Geometry: final body of the model. Coordinates: model frame, mm. Give positions to 0.01 mm unless a question says otherwise; leave off trailing zeros. Order: outer loops, then holes, each group sorted by start corner. A loop starts at its lowest first (then second) coordinate and runs counter-clockwise, first axis right, second up. Notation, with made-up numbers: (-20.75, -29.5) -> (34.25, -29.5) arc R8 ccw to (34.25, -20.5) -> close; hole circle Ø1 at (-1.5, 20.5). An arc over 180 degrees is marked (long way). One line per question, with ' | ' between items. Start each with the question number.
(1) Section C-C (z = 0.7). State how many separate pieces and enclosed holes the cut face has, then the cut area to 3 significant figures.
(2) Section A-A (y = 0). Return loops of the section in (x, z), then the cut area to 4 significant figures.
(3) Ray query, L1, parallel to Y at x = 0, z = -0.75; L2, parallel to X at y = -23.5, z = -1.15; L3, parallel to Y at x = -20, z = 0.9. Return the intervals inside material, ascending.
(4) First-contact query: pin 1 Ø6.5 at (x, y) = (-22.98, 22.98) entering from +Z; pin 2 Ø6.5 at (x, y) = (0, -45.75) entering from -Z; pin 3 Ø3 at (y, z) = (-35, 1.5) entering from +X. Flat tips, straight axial feed; report the tip coordinate or a pass-through.
(5) Section D-D (x = -15). Return loops of the section in (y, z), then the cut area to 3 significant figures.
```python
from build123d import *

# Parameters (mm, degrees)
SKETCH1_R           = 2.25
SKETCH1_R_2         = 22.5
BOSS_EXTRUDE1_DEPTH = 2.5
SKETCH3_R           = 4
CUT_EXTRUDE2_DEPTH  = 4
SKETCH4_R           = 4
CUT_EXTRUDE3_DEPTH  = 4


with BuildPart() as part:
    # Sketch1 → Boss-Extrude1 (new, symmetric)
    with BuildSketch(Plane.XY):
        with BuildLine():
            ThreePointArc((4.630966194, 47.635245902), (0, 50.75), (-4.630966194, 47.635245902))
            ThreePointArc((-4.630966194, 47.635245902), (-7.268500835, 43.914585958), (-11.283903543, 41.752078042))
            ThreePointArc((-11.283903543, 41.752078042), (-30.582368286, 30.582368286), (-41.752078042, 11.283903543))
            ThreePointArc((-41.752078042, 11.283903543), (-43.914585958, 7.268500835), (-47.635245902, 4.630966194))
            ThreePointArc((-47.635245902, 4.630966194), (-50.75, 0), (-47.635245902, -4.630966194))
            ThreePointArc((-47.635245902, -4.630966194), (-43.914585958, -7.268500835), (-41.752078042, -11.283903543))
            ThreePointArc((-41.752078042, -11.283903543), (-30.582368286, -30.582368286), (-11.283903543, -41.752078042))
            ThreePointArc((-11.283903543, -41.752078042), (-7.268500835, -43.914585958), (-4.630966194, -47.635245902))
            ThreePointArc((-4.630966194, -47.635245902), (0, -50.75), (4.630966194, -47.635245902))
            ThreePointArc((4.630966194, -47.635245902), (7.268500835, -43.914585958), (11.283903543, -41.752078042))
            ThreePointArc((11.283903543, -41.752078042), (30.582368286, -30.582368286), (41.752078042, -11.283903543))
            ThreePointArc((41.752078042, -11.283903543), (43.914585958, -7.268500835), (47.635245902, -4.630966194))
            ThreePointArc((47.635245902, -4.630966194), (50.75, 0), (47.635245902, 4.630966194))
            ThreePointArc((47.635245902, 4.630966194), (43.914585958, 7.268500835), (41.752078042, 11.283903543))
            ThreePointArc((41.752078042, 11.283903543), (30.582368286, 30.582368286), (11.283903543, 41.752078042))
            ThreePointArc((11.283903543, 41.752078042), (7.268500835, 43.914585958), (4.630966194, 47.635245902))
        make_face()
        with Locations((-45.75, 0)):
            Circle(SKETCH1_R, mode=Mode.SUBTRACT)
        with Locations((0, 45.75)):
            Circle(SKETCH1_R, mode=Mode.SUBTRACT)
        with Locations((45.75, 0)):
            Circle(SKETCH1_R, mode=Mode.SUBTRACT)
        with Locations((0, -45.75)):
            Circle(SKETCH1_R, mode=Mode.SUBTRACT)
        with Locations((-22.980970389, 22.980970389)):
            Circle(SKETCH1_R, mode=Mode.SUBTRACT)
        with Locations((22.980970389, 22.980970389)):
            Circle(SKETCH1_R, mode=Mode.SUBTRACT)
        with Locations((22.980970389, -22.980970389)):
            Circle(SKETCH1_R, mode=Mode.SUBTRACT)
        with Locations((-22.980970389, -22.980970389)):
            Circle(SKETCH1_R, mode=Mode.SUBTRACT)
        Circle(SKETCH1_R_2, mode=Mode.SUBTRACT)
    extrude(amount=BOSS_EXTRUDE1_DEPTH, both=True)

    # Sketch3 → Cut-Extrude2 (cut)
    with BuildSketch(Plane.XY.offset(2.5)):
        with Locations((-22.980970389, -22.980970389)):
            Circle(SKETCH3_R)
        with Locations((-22.980970389, 22.980970389)):
            Circle(SKETCH3_R)
        with Locations((22.980970389, 22.980970389)):
            Circle(SKETCH3_R)
        with Locations((22.980970389, -22.980970389)):
            Circle(SKETCH3_R)
    extrude(amount=-CUT_EXTRUDE2_DEPTH, mode=Mode.SUBTRACT)

    # Sketch4 → Cut-Extrude3 (cut)
    with BuildSketch(Plane(origin=(0, 0, -2.5), x_dir=(-1, 0, 0), z_dir=(0, 0, -1))):
        with Locations((0, 45.75)):
            Circle(SKETCH4_R)
        with Locations((45.75, 0)):
            Circle(SKETCH4_R)
        with Locations((0, -45.75)):
            Circle(SKETCH4_R)
        with Locations((-45.75, 0)):
            Circle(SKETCH4_R)
    extrude(amount=-CUT_EXTRUDE3_DEPTH, mode=Mode.SUBTRACT)


solid = part.part
```
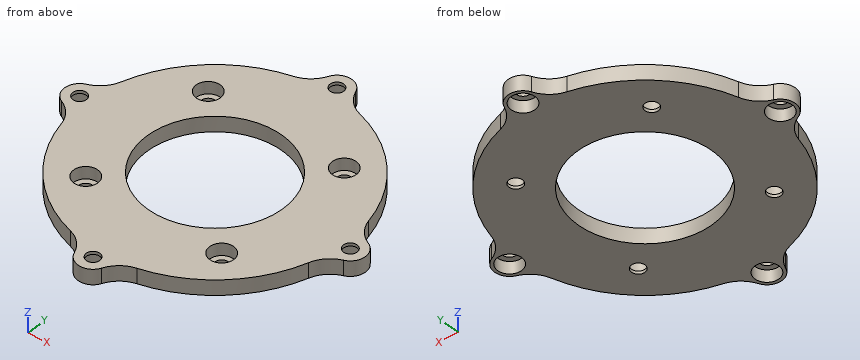
Response:
1) separate pieces: 1 | enclosed holes: 9 | area: 4,200 mm^2
2) outline: (-50.75, -2.5) -> (-49.75, -2.5) -> (-49.75, 1.5) -> (-48, 1.5) -> (-48, 2.5) -> (-50.75, 2.5) -> close; (-43.5, 1.5) -> (-41.75, 1.5) -> (-41.75, -2.5) -> (-22.5, -2.5) -> (-22.5, 2.5) -> (-43.5, 2.5) -> close; (22.5, -2.5) -> (41.75, -2.5) -> (41.75, 1.5) -> (43.5, 1.5) -> (43.5, 2.5) -> (22.5, 2.5) -> close; (48, 1.5) -> (49.75, 1.5) -> (49.75, -2.5) -> (50.75, -2.5) -> (50.75, 2.5) -> (48, 2.5) -> close | area: 209.5 mm^2
3) L1: y = -50.75 to -49.75, -41.75 to -22.5, 22.5 to 41.75, 49.75 to 50.75 | L2: x = -36.31 to -26.95, -19.01 to 19.01, 26.95 to 36.31 | L3: y = -38.35 to -25.65, -20.31 to -10.31, 10.31 to 20.31, 25.65 to 38.35
4) pin 1: stops at z = -1.5 | pin 2: stops at z = 1.5 | pin 3: stops at x = 27.36
5) outline: (-40.57, -2.5) -> (-16.77, -2.5) -> (-16.77, 2.5) -> (-40.57, 2.5) -> close; (16.77, -2.5) -> (40.57, -2.5) -> (40.57, 2.5) -> (16.77, 2.5) -> close | area: 238 mm^2
